Model file for the job. Use its own axes, mm. Round coordinates to 2 decimals unless told otherwise and drop trailing zeros. Order: outer loops, then holes, each group sorted by start corner. A loop starts at its lowest first (then second) coordinate and runs counter-clockwise, first axis right, second up. Notation, with made-up numbers: M 5,76 L 40,76 A10 ccw 40,84 Z; hole C 9.25,83.25 d4. An arc over 180 degrees is marked long. Return JSON: item names as keys, results as strings. Group by question number.
Item 1: Slice it at A-A on z = -3.75. Write the cut outline in (x, y), then the cut area to 3 significant figures.
Item 2: Slice it at B-B on z = 0.5. Give the number of separate pieces and of enclosed holes in the cut face, then the cut area to 3 significant figures.
Item 3: Probe line 1 along X through (y, z) = (2.35, -4); line 2 along X through (y, z) = (1.1, 0.75); line 3 along Z through (x, y) = (0.25, 0.65). List the from-to ranges inside material, lowest first.
Item 4: Pin check, flat tips, straight feed: pin 1 Ø1.5 at (x, z) = (0, -4) entering from -Y; pin 2 Ø1.5 at (y, z) = (1.5, 0.5) entering from +X. Stop position of each tip, or through.
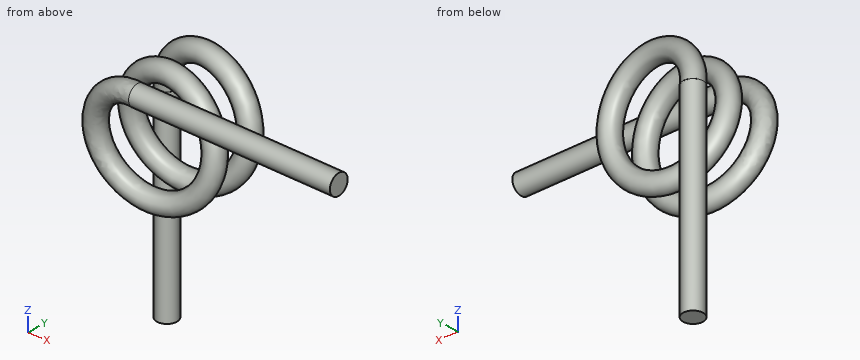
from build123d import *

# Parameters (mm, degrees)
SWEEP1_PITCH            = 1
SWEEP1_HEIGHT           = 2.5
SWEEP1_RADIUS           = 1.25
SWEEP1_START_ANGLE      = 90
SKETCH5_R               = 0.25
SKETCH6_R               = 0.25
BOSS_EXTRUDE1_DEPTH     = 5
CUT_EXTRUDE3_DEPTH      = 6.900213984
CUT_EXTRUDE3_DEPTH_BACK = 6.900213984
SKETCH11_R              = 0.25
BOSS_EXTRUDE3_DEPTH     = 5


with BuildPart() as part:
    # Sweep1: sweep along a helix
    with BuildLine() as sweep1_path:
        add(Helix(SWEEP1_PITCH, SWEEP1_HEIGHT, SWEEP1_RADIUS, center=(0, 0, 0), direction=(0, 1, 0), lefthand=True, mode=Mode.PRIVATE).rotate(Axis((0, 0, 0), (0, 1, 0)), SWEEP1_START_ANGLE))
    # Sketch5 → Sweep1 (sweep)
    with BuildSketch(Plane.XY):
        with Locations((-1.25, 2.5)):
            Circle(SKETCH5_R)
    sweep(path=sweep1_path.line, is_frenet=True)

    # Sketch6 → Boss-Extrude1 (add)
    with BuildSketch(Plane(origin=(0, 0, 0), x_dir=(-1, 0, 0), z_dir=(0, 0, -1))):
        with Locations(Location((1.249917128, 2.498189297, 0), (0, 0, 179.584887185))):
            Circle(SKETCH6_R)
    extrude(amount=BOSS_EXTRUDE1_DEPTH)

    # Sketch10 → Cut-Extrude3 (cut, two sides: drawn at the far end of the back side and taken through both)
    with BuildSketch(Plane.XY.offset(-CUT_EXTRUDE3_DEPTH_BACK)):
        Polygon((0, 0), (0, 0.476713955), (1.596533829, 0.476713955), (1.596533829, -0.338868321), (0, -0.310206334), align=None)
    extrude(amount=CUT_EXTRUDE3_DEPTH + CUT_EXTRUDE3_DEPTH_BACK, mode=Mode.SUBTRACT)

    # Sketch11 → Boss-Extrude3 (add)
    with BuildSketch(Plane(origin=(0, 0, 0), x_dir=(0, 0, -1), z_dir=(1, 0, 0))):
        with Locations(Location((-1.25, 0.25, 0), (0, 0, 65.074402292))):
            Circle(SKETCH11_R)
    extrude(amount=BOSS_EXTRUDE3_DEPTH)


solid = part.part
Output values:
{
 "1": {"outline": "C -1.25,2.5 d0.5", "area": "0.196 mm²"},
 "2": {"separate pieces": "5", "enclosed holes": "0", "area": "1.08 mm²"},
 "3": {"line 1": "-1.45 to -1.05", "line 2": "0.67 to 1.3", "line 3": "-1.44 to -1.01"},
 "4": {"pin 1": "through", "pin 2": "x = 1.5"}
}
